For this review, use the dimensioned drawing (mm, ordinates from the lowest corner) and the shaded views. Coordinates: 2 decimals unless noted, no trailing zeros. Order: outer loops, then holes, each group sorted by start corner. A loop starts at its lowest first (then second) coordinate and runs counter-clockwise, first axis right, second up. Notation, with made-up numbers: (54.25, -2) -> (91.25, -2) arc R30 cw to (91.25, 20) -> close; hole circle Ø11 at (-20.5, -33.5). An arc over 180 degrees is marked (long way). Return JSON: item names as keys, results as strings. Group by question number.
Item 1: Take a section at C-C (y = 14.5). Write out the cut boundary in (x, z), then the cut area to 3 significant figures.
Item 2: Take a section at B-B (x = 39). Write out the cut boundary in (y, z).
Item 3: For line 1 along Y through (x, z) = (18.5, 3.7); line 2 along X through (y, z) = (25, 4.05); line 3 along Z through (x, y) = (55.5, 34), list the stretches that pass through material, from the lowest coordinate up.
Item 4: Insertion check: pin 1 (0.8 mm diameter, centred on x = 24, z = 4, fed in from +Y); pin 2 (2 mm diameter, centred on x = 26.5, z = 2.5, fed in from +Y); pin 3 (1 mm diameter, centred on x = 24.5, y = 30.5, fed in from +Z); pin 4 (0.8 mm diameter, centred on y = 20, z = 3.5, fed in from -X). Each pin has a flat end and moves straight along its axis. Give the tip position at first contact, or say it passes through.
Item 5: Draft analysis for pull direction Y (two halves, no side actions). For the marked faces 1 and 2, state which applies: +Y half, -Y half, draft (parallel to the pull), parting line (faces both ways), or undercut.
Item 6: Take a section at A-A (z = 0.7). Write out the cut boundary in (x, y), then the cut area to 3 significant figures.
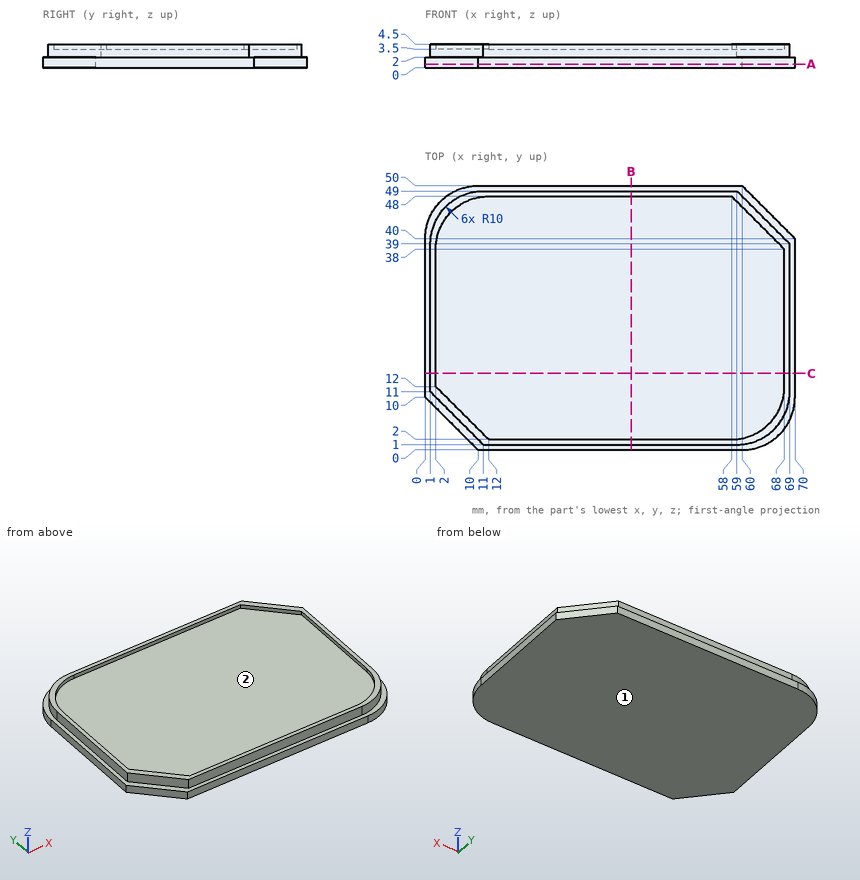
Findings below:
{
 "1": {"outline": "(0, 0) -> (70, 0) -> (70, 2) -> (69, 2) -> (69, 4.5) -> (68, 4.5) -> (68, 3.5) -> (2, 3.5) -> (2, 4.5) -> (1, 4.5) -> (1, 2) -> (0, 2) -> close", "area": "244 mm2"},
 "2": {"outline": "(0, 0) -> (50, 0) -> (50, 2) -> (49, 2) -> (49, 4.5) -> (48, 4.5) -> (48, 3.5) -> (2, 3.5) -> (2, 4.5) -> (1, 4.5) -> (1, 2) -> (0, 2) -> close"},
 "3": {"line 1": "y = 1 to 2, 48 to 49", "line 2": "x = 1 to 2, 68 to 69", "line 3": "z = 0 to 3.5"},
 "4": {"pin 1": "stops at y = 49", "pin 2": "stops at y = 50", "pin 3": "stops at z = 3.5", "pin 4": "stops at x = 1"},
 "5": {"face 1": "draft", "face 2": "undercut"},
 "6": {"outline": "(0, 10) -> (10, 0) -> (60, 0) arc R10 ccw to (70, 10) -> (70, 40) -> (60, 50) -> (10, 50) arc R10 ccw to (0, 40) -> close", "area": "3,360 mm2"}
}
